```python
from build123d import *

# Parameters (mm, degrees)
CROQUIS1_W              = 43
CROQUIS1_H              = 35
BRIDA_BASE1_DEPTH       = 1.5
CROQUIS6_W              = 59.566817112
CROQUIS6_H              = 45.88022185
CORTAR_EXTRUIR1_DEPTH   = 10
BRIDA_DE_ARISTA1_DEPTH  = 18
BRIDA_DE_ARISTA2_DEPTH  = 12
CORTAR_EXTRUIR2_DEPTH   = 10
SALIENTE_EXTRUIR1_DEPTH = 1.5
CORTAR_EXTRUIR3_DEPTH   = 10
BRIDA_DE_ARISTA3_DEPTH  = 15.985281374


# Sheet-metal steps are written as plain solids
with BuildPart() as part:
    # Croquis1 → Brida base1 (new body)
    with BuildSketch(Plane.XY):
        Rectangle(CROQUIS1_W, CROQUIS1_H)
    extrude(amount=-BRIDA_BASE1_DEPTH)

    # Croquis6 → Cortar-Extruir1 (cut)
    with BuildSketch(Plane.XY):
        Rectangle(CROQUIS6_W, CROQUIS6_H)
        Polygon((11, -17.5), (16.764888282, -13.45), (21.5, -13.45), (21.5, -1.45), (13.429731846, 9.247432799), (0, 17.5), (-14.121485549, 11.428046656), (-21.5, 4.5), (-21.5, -13.5), (-19.5, -17.5), align=None, mode=Mode.SUBTRACT)
    extrude(amount=-CORTAR_EXTRUIR1_DEPTH, mode=Mode.SUBTRACT)

    # Brida de arista1 section (across the edge) → Brida de arista1 (add)
    with BuildSketch(Plane(origin=(-22.2366, 4.5, 0), x_dir=(1, 0, 0), z_dir=(0, -1, 0))):
        with BuildLine():
            Line((-1.5, 0.7366), (-1.5, 6.5))
            Line((-1.5, 6.5), (0, 6.5))
            Line((0, 6.5), (0, 0.7366))
            ThreePointArc((0, 0.7366), (0.215745145, 0.215745145), (0.7366, 0))
            Line((0.7366, 0), (0.7366, -1.5))
            ThreePointArc((0.7366, -1.5), (-0.844915027, -0.844915027), (-1.5, 0.7366))
        make_face()
    extrude(amount=BRIDA_DE_ARISTA1_DEPTH)

    # Brida de arista2 section (across the edge) → Brida de arista2 (add)
    with BuildSketch(Plane(origin=(21.80510971, -13.45, 0), x_dir=(-0.7071067811865438, 0, 0.7071067811865512), z_dir=(0, 1, 0))):
        with BuildLine():
            Line((-1.5, 0.30510971), (-1.5, 20.378679656))
            Line((-1.5, 20.378679656), (0, 20.378679656))
            Line((0, 20.378679656), (0, 0.30510971))
            ThreePointArc((0, 0.30510971), (0.056070336, 0.023225094), (0.215745145, -0.215745145))
            Line((0.215745145, -0.215745145), (-0.844915027, -1.276405317))
            ThreePointArc((-0.844915027, -1.276405317), (-1.329748962, -0.550800055), (-1.5, 0.30510971))
        make_face()
    extrude(amount=BRIDA_DE_ARISTA2_DEPTH)

    # Croquis13 → Cortar-Extruir2 (cut)
    with BuildSketch(Plane(origin=(11.963215027, 0, -11.963215027), x_dir=(-0.7071067811865513, 0, -0.7071067811865438), z_dir=(0.7071067811865438, 0, -0.7071067811865513))):
        Polygon((-35.797220597, -1.45), (-23.797220597, -13.45), (-35.797220597, -13.45), align=None)
    extrude(amount=-CORTAR_EXTRUIR2_DEPTH, mode=Mode.SUBTRACT)

    # Croquis14 → Saliente-Extruir1 (add)
    with BuildSketch(Plane(origin=(11.963215027, 0, -11.963215027), x_dir=(-0.7071067811865513, 0, -0.7071067811865438), z_dir=(0.7071067811865438, 0, -0.7071067811865513))):
        Polygon((-35.797220597, -1.45), (-23.797220597, -1.45), (-30.161181628, 4.913961031), (-36.161181628, -1.086038969), align=None)
    extrude(amount=-SALIENTE_EXTRUIR1_DEPTH)

    # Croquis15 → Cortar-Extruir3 (cut)
    with BuildSketch(Plane(origin=(10.902554855, 0, -10.902554855), x_dir=(0.7071067811865513, 0, 0.7071067811865438), z_dir=(-0.7071067811865438, 0, 0.7071067811865513))):
        Polygon((30.161181628, 4.913961031), (36.161181628, -1.086038969), (35.100521456, -2.146699141), (29.100521456, 3.853300859), align=None)
    extrude(amount=-CORTAR_EXTRUIR3_DEPTH, mode=Mode.SUBTRACT)

    # Brida de arista3 section (across the edge) → Brida de arista3 (add)
    with BuildSketch(Plane(origin=(28.098030913, -13.970854855, 6.292921202), x_dir=(-0.5000000000000027, 0.7071067811865511, -0.4999999999999924), z_dir=(0.5000000000000054, 0.7071067811865441, 0.49999999999999967))):
        with BuildLine():
            Line((-1.5, 0.7366), (-1.5, 7.5))
            Line((-1.5, 7.5), (0, 7.5))
            Line((0, 7.5), (0, 0.7366))
            ThreePointArc((0, 0.7366), (0.215745145, 0.215745145), (0.7366, 0))
            Line((0.7366, 0), (0.7366, -1.5))
            ThreePointArc((0.7366, -1.5), (-0.844915027, -0.844915027), (-1.5, 0.7366))
        make_face()
    extrude(amount=BRIDA_DE_ARISTA3_DEPTH)


solid = part.part
```
The model under review builds one solid part; all positions refer to its coordinate system, in mm. A direction names the side the tool comes from. Give positions to 0.01 mm unless a question says otherwise; leave off trailing zeros. Write each loop counter-clockwise with the first axis right and the second up, starting at its lowest first coordinate (ties: lowest second). Pieces come first, ordered by that corner, then holes. Notation, with made-up numbers: (12.5, -36) -> (21.5, -36) arc R14 cw to (21.5, -15) -> close; hole circle Ø6 at (-36.5, 34). An arc over 180 degrees is marked (long way). Put each result on its own line as item: value.
(1) The part is to be moulded in two halves that separate along X. For faces 1 (the flat face through (13.842, -15.503, -0.74)), 2 (the flat face through (-23, -4, 6.5)), 3 (the flat face through (0, -4, 0)), say which applies: pulls with the +X half, pulls with the -X half, needs draft (parallel to the pull), parting line crosses it, or undercut.
Results are:
face 1: pulls with the +X half
face 2: needs draft
face 3: undercut
(2) We need section A-A, the plane y = -0.5. Give the boundary of the cut face in (x, z), and give its area (3 significant figures).
Results are:
outline: (-23.74, 0.74) arc R2.24 ccw to (-21.5, -1.5) -> (20.78, -1.5) -> (20.78, 0) -> (-21.5, 0) arc R0.74 cw to (-22.24, 0.74) -> (-22.24, 6.5) -> (-23.74, 6.5) -> close; (28.4, 6.6) -> (29.46, 5.54) -> (35.62, 11.69) -> (34.56, 12.75) -> close
area: 88.6 mm²
(3) For pin 1 Ø10.5 at (x, y) = (9.5, 5) entering from +Z; pin 2 Ø6.5 at (y, z) = (-6.5, 4.5) entering from +X; pin 3 Ø1.6 at (x, y) = (-22.5, -7.5) entering from +Z; pin 4 Ø12 at (x, z) = (-4, 9) entering from -Y, all flat-tipped, find the tip position at first contact; note any pin that passes through.
Results are:
pin 1: z = 0
pin 2: x = 31.68
pin 3: z = 6.5
pin 4: through
(4) We need section D-D, the plane z = 17.75. Give the boundary of the cut face in (x, y).
Results are:
outline: (28.95, -7.39) -> (34.13, -3.73) -> (32.63, -2.67) -> (28.95, -5.27) -> close
(5) We need section B-B, the plane z = 2. Give the boundary of the cut face in (x, y), and give its area (3 significant figures).
Results are:
outline: (-23.74, -13.5) -> (-22.24, -13.5) -> (-22.24, 4.5) -> (-23.74, 4.5) -> close; (23.81, -13.45) -> (25.93, -13.45) -> (25.93, -1.45) -> (23.81, -1.45) -> close
area: 52.5 mm²
(6) Tool access review of faces 4 (the flat face through (27.445, -6.6, 5.64)), 5 (the flat face through (-23.737, -4, 4)), 6 (the flat face through (30.116, 1.165, 7.236)): name each direction out of +Z, -Z, +X, -X, +Y, -Y from which nothing blocks a thin tool from reaching the whole face with its end or side.
Results are:
face 4: +Y
face 5: +Z, -Z, -X, +Y, -Y
face 6: -Z, +Y
(7) To check wall thickness, follow probe 1 along Z at (x, y) = (-4, 9); probe 2 along X at (y, z) = (-2.5, 0.5); probe 3 along X at (y, z) = (4, 1.5). State the ranges of each line that lie inside material, in increasing order. Write a range as from..to.
Results are:
probe 1: -1.5..0
probe 2: -23.72..-22.2, 22.31..24.43
probe 3: -23.74..-22.24
(8) We need section C-C, the plane y = 10. Give the boundary of the cut face in (x, z).
Results are:
outline: (-15.64, -1.5) -> (12.21, -1.5) -> (12.21, 0) -> (-15.64, 0) -> close
